For this review, take the finished solid that the model builds, in its own axes (mm). A direction names the side the tool comes from. Round coordinates to 2 decimals unless told otherwise and drop trailing zeros. Write each loop counter-clockwise with the first axis right and the second up, starting at its lowest first coordinate (ties: lowest second). Pieces come first, ordered by that corner, then holes. Notation, with made-up numbers: M 18,0.5 L 44,0.5 A7 ccw 44,11.5 Z; hole C -28.5,-40 d4. An arc over 180 degrees is marked long. Write each question's results on one line, items separated by ' | '. Start each with the question number.
```python
from build123d import *

# Parameters (mm, degrees)
SKETCH2_R               = 11
BOSS_EXTRUDE1_DEPTH     = 40
CUT_EXTRUDE1_DEPTH      = 61.695963622
CUT_EXTRUDE1_DEPTH_BACK = 61.695963622
SKETCH3_W               = 44
SKETCH3_H               = 40
SKETCH4_R               = 5.5
BOSS_EXTRUDE2_DEPTH     = 25
BOSS_EXTRUDE2_TAPER     = 5


with BuildPart() as part:
    # Sketch2 → Boss-Extrude1 (new, symmetric)
    with BuildSketch(Plane.XY):
        with BuildLine():
            Line((0, 22), (-40, 22))
            Line((-40, 22), (-40, -22))
            Line((-40, -22), (0, -22))
            ThreePointArc((0, -22), (22, 0), (0, 22))
        make_face()
        Circle(SKETCH2_R, mode=Mode.SUBTRACT)
    extrude(amount=BOSS_EXTRUDE1_DEPTH, both=True)

    # Sketch3 → Cut-Extrude1 (cut, two sides: drawn at the far end of the back side and taken through both)
    with BuildSketch(Plane(origin=(0, 0, 0), x_dir=(1, 0, 0), z_dir=(0, 1, 0)).offset(-CUT_EXTRUDE1_DEPTH_BACK)):
        Rectangle(SKETCH3_W, SKETCH3_H)
    extrude(amount=CUT_EXTRUDE1_DEPTH + CUT_EXTRUDE1_DEPTH_BACK, mode=Mode.SUBTRACT)

    # Sketch4 → Boss-Extrude2 (add)
    with BuildSketch(Plane.ZY.offset(40)):
        Circle(SKETCH4_R)
    extrude(amount=BOSS_EXTRUDE2_DEPTH, taper=BOSS_EXTRUDE2_TAPER)


solid = part.part
```
Item 1: We need section A-A on x = 4.5. State the section outline as (y, z) points, then the cut area to 3 significant figures.
Item 2: We need section C-C on y = -19. State the section outline as (x, z) points, then the cut area to 3 significant figures.
Item 3: Mouldability with a two-part tool opening along Z and no side actions: class faces 1 (the flat face through (-40, 0, 9)), 2 (the conical face through (-52.675, 1.319, 4.188)), 3 (the flat face through (-10, -5, 20)) as pulls with the +Z half, pulls with the -Z half, needs draft (parallel to the pull), parting line crosses it, or undercut.
Item 4: For probe 1 along X at (y, z) = (0, -35.25); probe 2 along Y at (x, z) = (0, 28.25); probe 3 along Z at (x, y) = (14, -2), list the stretches that pass through material, from the lowest coordinate up.
Item 5: We need section B-B on z = 26.5. State the section outline as (x, y) points.
Item 6: Insertion check: P1, Ø4, axis at y = 4, z = -15.5, coming from the -X side. The pin has a flat end and moves straight along its axis. Give the tip position at first contact, or say it passes through.
Item 7: We need section D-D on z = 0. State the section outline as (x, y) points.
Item 8: For faces 4 (the flat face through (-25, -22, 1)), 5 (the flat face through (-10, -5, -20)), list the 3-axis set-ups (+Z, -Z, +X, -X, +Y, -Y) from which the entire face can be reached by the end or side of a thin tool; tool diameter is ignored.
Numbers:
1) outline: M -21.53,-40 L -10.04,-40 L -10.04,-20 L -21.53,-20 Z; M -21.53,20 L -10.04,20 L -10.04,40 L -21.53,40 Z; M 10.04,-40 L 21.53,-40 L 21.53,-20 L 10.04,-20 Z; M 10.04,20 L 21.53,20 L 21.53,40 L 10.04,40 Z | area: 920 mm^2
2) outline: M -40,-40 L 11.09,-40 L 11.09,-20 L -22,-20 L -22,20 L 11.09,20 L 11.09,40 L -40,40 Z | area: 2,760 mm^2
3) face 1: needs draft | face 2: parting line crosses it | face 3: undercut
4) probe 1: x = -40 to -11, 11 to 22 | probe 2: y = -22 to -11, 11 to 22 | probe 3: z = -40 to -20, 20 to 40
5) outline: M -40,-22 L 0,-22 A22 ccw 0,22 L -40,22 Z; hole C 0,0 d22
6) P1: stops at x = -40
7) outline: M -65,-3.31 L -40,-5.5 L -40,-22 L -22,-22 L -22,22 L -40,22 L -40,5.5 L -65,3.31 Z
8) face 4: +Z, -Z, +X, -X, -Y | face 5: +X, +Y, -Y
